CAD build for the part. Positions are in the model's coordinates, mm. A direction names the side the tool comes from. Coordinates: 2 decimals unless noted, no trailing zeros. Write each loop counter-clockwise with the first axis right and the second up, starting at its lowest first coordinate (ties: lowest second). Pieces come first, ordered by that corner, then holes. Notation, with made-up numbers: (-24, -36) - (26, -36) arc R16 cw to (26, -29) - close; hole circle Ø9 at (-32.5, 89). An arc over 180 degrees is marked (long way). Answer in a Markdown table with one row per item. Add a question column.
Q1. 3-axis set-ups, long thin cutter, end or side, ignore diameter. For faces 1 (the cylindrical face through (40.49, -40.65, 38.84)), 2 (the conical face through (-22.61, -54.93, 60.56)), 3 (the cylindrical face through (-49.23, -48.88, 31.06)): which of +Z, -Z, +X, -X, +Y, -Y reach the whole face in a straight line?
Q2. Drill centre lines: line 1 along Y through (x, z) = (-33.5, 16.5); line 2 along Z through (x, y) = (36, -4). Where is each one in solid material? Low to high. Write a range as from..to.
Q3. Band-saw the part on D-D (z = 40). List the corners of the cut face in (x, y), and give its area (3 significant figures).
Q4. Two-plate mould, pull along Y, no slides. Class faces 4 (the cylindrical face through (48.88, -49.23, 31.06)), 5 (the cylindrical face through (49.23, 48.88, 31.06)), 6 (the cylindrical face through (40.65, 40.49, 38.84)): +Y half, -Y half, draft (parallel to the pull), parting line (faces both ways), or undercut.
Q5. Pin check, flat tips, straight feed: pin 1 (3 mm diameter, centred on x = -12, z = 22.5, fed in from -Y); pin 2 (9 mm diameter, centred on y = -51, z = 34, fed in from -X); pin 3 (4 mm diameter, centred on x = 4, y = -48, fed in from +Z). Stop position of each tip, or through.
Q6. Band-saw the part on B-B (y = -15.5). List the corners of the cut face in (x, z), and give its area (3 significant figures).
Q7. Band-saw the part on A-A (z = 7.5). List the corners of the cut face in (x, y), and give its area (3 significant figures).
```python
from build123d import *

# Parameters (mm, degrees)
F1_DEPTH = 65
F3_DEPTH = 53
F5_DEPTH = 12
F6_SIZE  = 1.99999


# Not quite as in the source:
# - a fillet or chamfer is up to 0.001 mm smaller than in the source, because OpenCascade refuses the exact size


with BuildPart() as f1:
    # F0 (on Top) → F1 (new body)
    with BuildSketch(Plane.XY):
        with BuildLine():
            Line((55.5, -33.5), (55.5, 33.5))
            ThreePointArc((55.5, 33.5), (49.0563491861, 49.0563491861), (33.5, 55.5))
            Line((33.5, 55.5), (-33.5, 55.5))
            ThreePointArc((-33.5, 55.5), (-49.0563491861, 49.0563491861), (-55.5, 33.5))
            Line((-55.5, 33.5), (-55.5, -33.5))
            ThreePointArc((-55.5, -33.5), (-49.0563491861, -49.0563491861), (-33.5, -55.5))
            Line((-33.5, -55.5), (33.5, -55.5))
            ThreePointArc((33.5, -55.5), (49.0563491861, -49.0563491861), (55.5, -33.5))
        make_face()
    extrude(amount=F1_DEPTH)

    # F2 (on face) → F3 (cut, through all)
    with BuildSketch(Plane.XY.offset(65)):
        with BuildLine():
            Line((33.5, 43.5), (-33.5, 43.5))
            ThreePointArc((-33.5, 43.5), (-40.5710678119, 40.5710678119), (-43.5, 33.5))
            Line((-43.5, 33.5), (-43.5, -33.5))
            ThreePointArc((-43.5, -33.5), (-40.5710678119, -40.5710678119), (-33.5, -43.5))
            Line((-33.5, -43.5), (33.5, -43.5))
            ThreePointArc((33.5, -43.5), (40.5710678119, -40.5710678119), (43.5, -33.5))
            Line((43.5, -33.5), (43.5, 33.5))
            ThreePointArc((43.5, 33.5), (40.5710678119, 40.5710678119), (33.5, 43.5))
        make_face()
    extrude(amount=-F3_DEPTH, mode=Mode.SUBTRACT)

    # F4 (on face) → F5 (cut, through all)
    with BuildSketch(Plane.XZ.offset(55.5)):
        with BuildLine():
            ThreePointArc((-30, 65), (-21.5147186258, 61.4852813742), (-18, 53))
            Line((-18, 53), (-18, 26))
            ThreePointArc((-18, 26), (-15.0710678119, 18.9289321881), (-8, 16))
            Line((-8, 16), (8, 16))
            ThreePointArc((8, 16), (15.0710678119, 18.9289321881), (18, 26))
            Line((18, 26), (18, 53))
            ThreePointArc((18, 53), (21.5147186258, 61.4852813742), (30, 65))
            Line((30, 65), (-30, 65))
        make_face()
    extrude(amount=-F5_DEPTH, mode=Mode.SUBTRACT)

    # F6 (size 2 in the source; OpenCascade refuses exactly that, so slightly less here)
    f6_edges = [f1.edges().sort_by_distance(p)[0] for p in [
        (55.5, 0, 65),
        (-43.5, 0, 65),
        (0, 43.5, 12),
        (-40.571068, 40.571068, 12),
        (-43.5, 0, 12),
        (-40.571068, -40.571068, 12),
        (0, -43.5, 12),
        (40.571068, -40.571068, 12),
        (43.5, 0, 12),
        (40.571068, 40.571068, 12),
    ]]
    chamfer(f6_edges, length=F6_SIZE)


solid = f1.part
```
Checked values:
| question | item | result |
|---|---|---|
| 1 | face 1 | +Z |
| 1 | face 2 | +Z, -Y |
| 1 | face 3 | +Z, -Z, -X, -Y |
| 2 | line 1 | y = -55.5..-43.5, 43.5..55.5 |
| 2 | line 2 | z = 0..12 |
| 3 | outline | (-55.5, -33.5) arc R22 ccw to (-33.5, -55.5) - (-20, -55.5) - (-18, -53.5) - (-18, -45.5) - (-20, -43.5) - (-33.5, -43.5) arc R10 cw to (-43.5, -33.5) - (-43.5, 33.5) arc R10 cw to (-33.5, 43.5) - (33.5, 43.5) arc R10 cw to (43.5, 33.5) - (43.5, -33.5) arc R10 cw to (33.5, -43.5) - (20, -43.5) - (18, -45.5) - (18, -53.5) - (20, -55.5) - (33.5, -55.5) arc R22 ccw to (55.5, -33.5) - (55.5, 33.5) arc R22 ccw to (33.5, 55.5) - (-33.5, 55.5) arc R22 ccw to (-55.5, 33.5) - close |
| 3 | area | 3,980 mm² |
| 4 | face 4 | -Y half |
| 4 | face 5 | +Y half |
| 4 | face 6 | undercut |
| 5 | pin 1 | stops at y = 43.5 |
| 5 | pin 2 | stops at x = -51.25 |
| 5 | pin 3 | stops at z = 16 |
| 6 | outline | (-55.5, 0) - (55.5, 0) - (55.5, 63) - (53.5, 65) - (45.5, 65) - (43.5, 63) - (43.5, 14) - (41.5, 12) - (-41.5, 12) - (-43.5, 14) - (-43.5, 63) - (-45.5, 65) - (-53.5, 65) - (-55.5, 63) - close |
| 6 | area | 2,600 mm² |
| 7 | outline | (-55.5, -33.5) arc R22 ccw to (-33.5, -55.5) - (33.5, -55.5) arc R22 ccw to (55.5, -33.5) - (55.5, 33.5) arc R22 ccw to (33.5, 55.5) - (-33.5, 55.5) arc R22 ccw to (-55.5, 33.5) - close |
| 7 | area | 11,900 mm² |
